```python
from build123d import *

# Parameters (mm, degrees)
F0_W     = 20
F0_H     = 20
F0_R     = 2.375
F1_DEPTH = 4.5
F3_DEPTH = 5
F4_R     = 2.375
F5_DEPTH = 3


with BuildPart() as f1:
    # F0 (on Front) → F1 (new body)
    with BuildSketch(Plane.XZ):
        with Locations((2.156144, 3.828467)):
            Rectangle(F0_W, F0_H)
        with Locations((2.156144, 3.828467)):
            Circle(F0_R, mode=Mode.SUBTRACT)
    extrude(amount=F1_DEPTH)

    # F2 (on face) → F3 (join)
    with BuildSketch(Plane.XZ.offset(4.5)):
        Polygon((-5.343856, 13.828467), (-7.843856, 13.828467), (-7.843856, -6.171533), (12.156144, -6.171533), (12.156144, -3.671533), (-5.343856, -3.671533), align=None)
    extrude(amount=F3_DEPTH)

    # F4 (on face) → F5 (cut)
    with BuildSketch(Plane.XZ.offset(4.5)):
        Polygon((0.077683, 7.428467), (-2.000778, 3.828467), (0.077683, 0.228467), (4.234605, 0.228467), (6.313066, 3.828467), (4.234605, 7.428467), align=None)
        with Locations((2.156144, 3.828467)):
            Circle(F4_R, mode=Mode.SUBTRACT)
    extrude(amount=-F5_DEPTH, mode=Mode.SUBTRACT)


solid = f1.part
```
Could you check a few things on this model? Use its own coordinates, in mm. A direction names the side the tool comes from. Round coordinates to 2 decimals unless told otherwise and drop trailing zeros. Write each loop counter-clockwise with the first axis right and the second up, starting at its lowest first coordinate (ties: lowest second). Pieces come first, ordered by that corner, then holes.
(1) Thinking about a two-plate mould opening in X: for faces 1 (the face through (12.156, -3, 4)), 2 (the face through (2, -3, 13.828)), 3 (the face through (3, -1.5, 6.3)), which applies, +X half, -X half, draft (parallel to the pull), parting line (faces both ways), or undercut?
Findings below:
face 1: +X half
face 2: draft
face 3: undercut
(2) Suppose I cut it at C-C on x = 3.75. Write out the boundary of the cut face in (y, z), and give its area (3 significant figures).
Findings below:
outline: (-9.5, -6.17) - (0, -6.17) - (0, 2.07) - (-1.5, 2.07) - (-1.5, 0.23) - (-4.5, 0.23) - (-4.5, -3.67) - (-9.5, -3.67) - close; (-4.5, 7.43) - (-1.5, 7.43) - (-1.5, 5.59) - (0, 5.59) - (0, 13.83) - (-4.5, 13.83) - close
area: 75.6 mm2
(3) Which directions (+Z, -Z, +X, -X, +Y, -Y) give clear straight access to the entire face, cutting with the end or side of a thin tool? Please do faces 4 (the face through (2, -3, 7.428)), 5 (the face through (-2, -9.5, -4)), 6 (the face through (-5.344, -7, 5)).
Findings below:
face 4: -Y
face 5: +Z, -Z, +X, -X, -Y
face 6: +Z, +X, -Y
(4) For pin 1 (4 mm diameter, centred on y = -7, z = 5.5, fed in from +X); pin 2 (3.5 mm diameter, centred on x = 1, z = 5, fed in from -Y), each with a flat end and sliding along its axis, tell me the tip position at first contact or that it passes through.
Findings below:
pin 1: stops at x = -5.34
pin 2: stops at y = -1.5
(5) Suppose I cut it at A-A on z = 3. Write out the boundary of the cut face in (x, y), and give its area (3 significant figures).
Findings below:
outline: (-7.84, -9.5) - (-5.34, -9.5) - (-5.34, -4.5) - (-1.52, -4.5) - (-1.52, -1.5) - (-0.07, -1.5) - (-0.07, 0) - (-7.84, 0) - close; (4.38, -1.5) - (5.83, -1.5) - (5.83, -4.5) - (12.16, -4.5) - (12.16, 0) - (4.38, 0) - close
area: 73.8 mm2
(6) If I drill on probe 1 along X at (y, z) = (-4.75, 0); probe 2 along Y at (x, z) = (8.25, 3); probe 3 along Z at (x, y) = (9, -8.75), over which ranges is the centre line in solid material (lowest first)?
Findings below:
probe 1: x = -7.84 to -5.34
probe 2: y = -4.5 to 0
probe 3: z = -6.17 to -3.67
(7) Suppose I cut it at B-B on y = -0.75. Write out the boundary of the cut face in (x, z) (3 decimals).
Findings below:
outline: (-7.844, -6.172) - (12.156, -6.172) - (12.156, 13.828) - (-7.844, 13.828) - close; hole circle Ø4.75 at (2.156, 3.828)
(8) Suppose I cut it at D-D on x = 8.75. Write out the boundary of the cut face in (y, z).
Findings below:
outline: (-9.5, -6.17) - (0, -6.17) - (0, 13.83) - (-4.5, 13.83) - (-4.5, -3.67) - (-9.5, -3.67) - close
